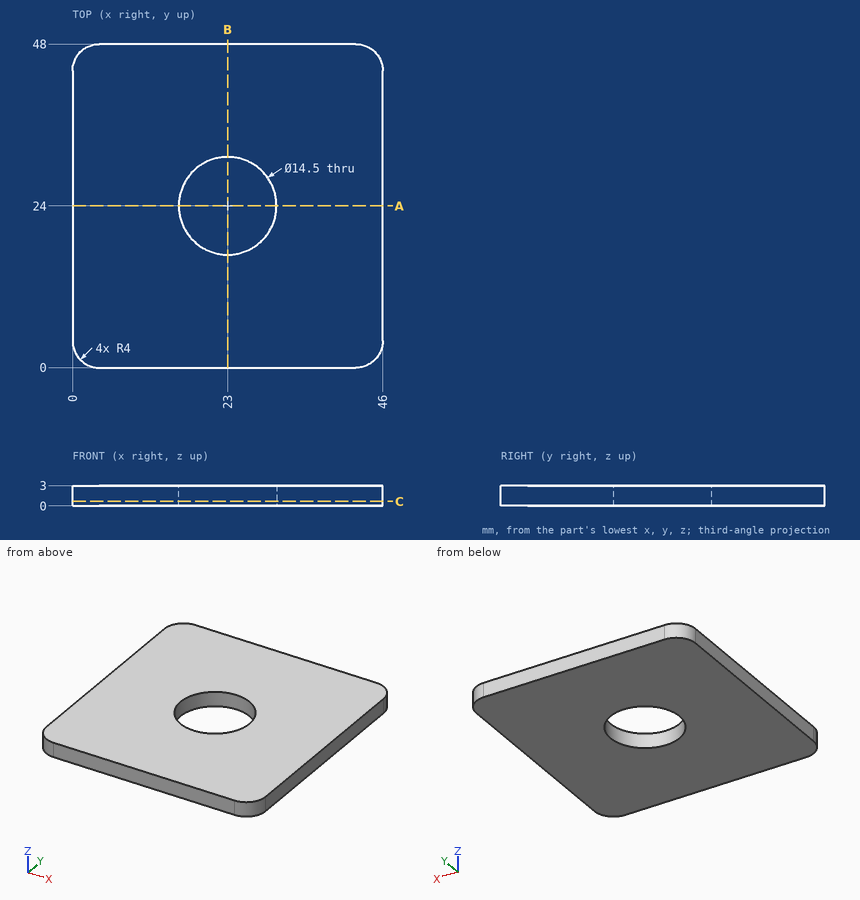
For this review, use the dimensioned drawing (mm, ordinates from the lowest corner) and the shaded views. Give positions to 0.01 mm unless a question says otherwise; leave off trailing zeros. Order: outer loops, then holes, each group sorted by start corner. A loop starts at its lowest first (then second) coordinate and runs counter-clockwise, first axis right, second up. Notation, with made-up numbers: (7, 13) - (64, 13) arc R8 cw to (64, 27) - close; hole circle Ø10 at (46.5, -31). An arc over 180 degrees is marked (long way). Write item = value, one per line. Start each with the question number.
Q1. We need section A-A on y = 24. State the section outline as (x, z) points, plus the area to 3 significant figures.
Q2. To check wall thickness, follow L1, parallel to Y at x = 23, z = 1.95; L2, parallel to X at y = 29, z = 1.4; L3, parallel to Y at x = 21.5, z = 1.7. State the ranges of each line that lie inside material, in increasing order. Write a range as from..to.
Q3. We need section C-C on z = 0.7. State the section outline as (x, y) points.
Q4. We need section B-B on x = 23. State the section outline as (y, z) points, plus the area to 4 significant figures.
Working result:
q1.outline = (0, 0) - (15.75, 0) - (15.75, 3) - (0, 3) - close; (30.25, 0) - (46, 0) - (46, 3) - (30.25, 3) - close
q1.area = 94.5 mm²
q2.L1 = 0..16.75, 31.25..48
q2.L2 = 0..17.75, 28.25..46
q2.L3 = 0..16.91, 31.09..48
q3.outline = (0, 4) arc R4 ccw to (4, 0) - (42, 0) arc R4 ccw to (46, 4) - (46, 44) arc R4 ccw to (42, 48) - (4, 48) arc R4 ccw to (0, 44) - close; hole circle Ø14.5 at (23, 24)
q4.outline = (0, 0) - (16.75, 0) - (16.75, 3) - (0, 3) - close; (31.25, 0) - (48, 0) - (48, 3) - (31.25, 3) - close
q4.area = 100.5 mm²
